The listing builds one solid part. Answer for the finished solid, in the listing's coordinates (mm). A direction names the side the tool comes from. Round coordinates to 2 decimals unless told otherwise and drop trailing zeros. Write each loop counter-clockwise with the first axis right and the second up, starting at its lowest first coordinate (ties: lowest second). Pieces come first, ordered by that corner, then holes. Notation, with made-up numbers: (88, 73.25) - (125, 73.25) arc R21 ccw to (125, 90.25) - close; hole circle Ø1 at (73.25, 44). An arc over 180 degrees is marked (long way). Return JSON: item names as keys, results as strings. Group by question number.
(1) Find the intervals of material crossed by line 1 along Y through (x, z) = (15, 8.25); line 2 along Y through (x, z) = (0, -0.15) (3 decimals); line 3 along Z through (x, y) = (-8.5, 4.25), in increasing order. Write a range as [from, to].
(2) Which of the six approach directions +Z, -Z, +X, -X, +Y, -Y give full straight-line access (tool end or side, diameter ignored) to faces 1 (the cylindrical face through (1.717, -0.541, -0.419)), 2 (the flat face through (9, 7, 0.5)), 3 (the flat face through (-15, 5, -0.001)), 4 (the flat face through (14.5, -5.5, 3.5))?
(3) Each of these flat-tipped pins is pushed along its axis until it touches: pin 1 (6 mm diameter, centred on x = 6, z = 6, fed in from +Y); pin 2 (4 mm diameter, centred on x = 0, y = -0.5, fed in from -Z); pin 3 (6 mm diameter, centred on y = 7.5, z = 0, fed in from +X); pin 4 (1.5 mm diameter, centred on x = -7.5, y = 1, fed in from +Z). Where does it stop, or does it pass through?
(4) Determine the mould class of faces 5 (the flat face through (11, 9, 1)), 6 (the cylindrical face through (1.25, -0.96, 0.59)), 7 (the flat face through (0, 8, 2)) for opening direction X: +X half, -X half, draft (parallel to the pull), parting line (faces both ways), or undercut.
(5) Section A-A, the plane z = 5.25 is taken. Write down the section's boundary in (x, y), then the cut area to 3 significant figures.
(6) Section C-C, the plane x = -13 is taken. Write down the section's boundary in (y, z) (3 decimals), then the cut area to 3 significant figures.
(7) Section B-B, the plane y = 0 is taken. Write down the section's boundary in (x, z) (3 decimals), then the cut area to 3 significant figures.
```python
from build123d import *

# Parameters (mm, degrees)
BOSS_EXTRUDE1_DEPTH     = 2
SKETCH2_R               = 1.575
BOSS_EXTRUDE2_DEPTH     = 4
SKETCH3_R               = 1.8
BOSS_EXTRUDE3_DEPTH     = 0.85
SKETCH4_W               = 2
SKETCH4_H               = 17
BOSS_EXTRUDE4_DEPTH     = 0.001
SKETCH5_W               = 18
SKETCH5_H               = 2
BOSS_EXTRUDE5_DEPTH     = 0.001
SKETCH6_W               = 2.001
SKETCH6_H               = 2
BOSS_EXTRUDE6_DEPTH     = 5
BOSS_EXTRUDE7_DEPTH     = 0.001
CUT_EXTRUDE1_DEPTH      = 20.519323784
SKETCH9_W               = 2.937742252
SKETCH9_H               = 8
CUT_EXTRUDE2_DEPTH      = 0.001
CUT_EXTRUDE11_START     = -0.001
SKETCH21_R              = 9.75
SKETCH21_R_2            = 1.8
CUT_EXTRUDE11_DEPTH     = 0.001
SKETCH10_W              = 32
SKETCH10_H              = 2
BOSS_EXTRUDE8_DEPTH     = 7
FILLET1_R               = 0.5
SKETCH11_R              = 0.625
BOSS_EXTRUDE9_DEPTH     = 2
SKETCH14_W              = 2
SKETCH14_H              = 2
CUT_EXTRUDE5_DEPTH      = 22.401355237
SKETCH12_R              = 0.675
CUT_EXTRUDE3_DEPTH      = 2.5
CUT_EXTRUDE6_DEPTH      = 2
FILLET2_R               = 0.5
FILLET3_R               = 0.5
FILLET4_R               = 2
CUT_EXTRUDE7_DEPTH      = 26.019992106
CUT_EXTRUDE7_DEPTH_BACK = 1
SKETCH19_R              = 0.625
CUT_EXTRUDE9_DEPTH      = 2


with BuildPart() as part:
    # Sketch1 → Boss-Extrude1 (new body)
    with BuildSketch(Plane.XY):
        Polygon((-11, 6), (-11, 11), (11, 11), (11, 6), (11, -6), (-11, -6), align=None)
    extrude(amount=BOSS_EXTRUDE1_DEPTH)

    # Sketch3 → Boss-Extrude3 (add)
    with BuildSketch(Plane(origin=(0, 0, 0), x_dir=(-1, 0, 0), z_dir=(0, 0, -1))):
        with Locations(Location((0, 0, 0), (0, 0, 180))):
            Circle(SKETCH3_R)
    extrude(amount=BOSS_EXTRUDE3_DEPTH)

    # Sketch4 → Boss-Extrude4 (add)
    with BuildSketch(Plane(origin=(0, 0, 0), x_dir=(-1, 0, 0), z_dir=(0, 0, -1))):
        with Locations((10, 2.5)):
            Rectangle(SKETCH4_W, SKETCH4_H)
        with Locations((-10, 2.5)):
            Rectangle(SKETCH4_W, SKETCH4_H)
    extrude(amount=BOSS_EXTRUDE4_DEPTH)

    # Sketch5 → Boss-Extrude5 (add)
    with BuildSketch(Plane(origin=(0, 0, 0), x_dir=(-1, 0, 0), z_dir=(0, 0, -1))):
        with Locations((0, 10)):
            Rectangle(SKETCH5_W, SKETCH5_H)
    extrude(amount=BOSS_EXTRUDE5_DEPTH)

    # Sketch6 → Boss-Extrude6 (add)
    with BuildSketch(Plane(origin=(11, 0, 0), x_dir=(0, 0, -1), z_dir=(1, 0, 0))):
        with Locations((-0.9995, -5)):
            Rectangle(SKETCH6_W, SKETCH6_H)
        with Locations((-0.9995, 5)):
            Rectangle(SKETCH6_W, SKETCH6_H)
    boss_extrude6 = extrude(amount=BOSS_EXTRUDE6_DEPTH)

    # Mirror1: Boss-Extrude6 across plane
    add(boss_extrude6.mirror(Plane(origin=(0, 0, 0), x_dir=(0, 0, 1), z_dir=(1, 0, 0))))

    # Sketch7 → Boss-Extrude7 (add)
    with BuildSketch(Plane(origin=(0, 0, -0.001), x_dir=(-1, 0, 0), z_dir=(0, 0, -1))):
        with BuildLine():
            ThreePointArc((-6.708203932, -6), (-8.407551231, -3.211398808), (-9, 0))
            Line((-9, 0), (-9, -6))
            Line((-9, -6), (-6.708203932, -6))
        make_face()
        with BuildLine():
            Line((-9, 9), (-9, 0))
            ThreePointArc((-9, 0), (-6.363961031, 6.363961031), (0, 9))
            Line((0, 9), (-9, 9))
        make_face()
    boss_extrude7 = extrude(amount=-BOSS_EXTRUDE7_DEPTH)

    # Sketch8 → Cut-Extrude1 (cut, through all)
    with BuildSketch(Plane(origin=(0, 0, -0.001), x_dir=(-1, 0, 0), z_dir=(0, 0, -1))):
        with BuildLine():
            Line((-11, 4), (-9.16515139, 4))
            ThreePointArc((-9.16515139, 4), (-10, 0), (-9.16515139, -4))
            Line((-9.16515139, -4), (-11, -4))
            Line((-11, -4), (-11, 4))
        make_face()
    cut_extrude1 = extrude(amount=-CUT_EXTRUDE1_DEPTH, mode=Mode.SUBTRACT)

    # Sketch9 → Cut-Extrude2 (cut)
    with BuildSketch(Plane(origin=(0, 0, -0.001), x_dir=(-1, 0, 0), z_dir=(0, 0, -1))):
        with Locations((-9.531128874, 0)):
            Rectangle(SKETCH9_W, SKETCH9_H)
    cut_extrude2 = extrude(amount=-CUT_EXTRUDE2_DEPTH, mode=Mode.SUBTRACT)

    # Mirror2: Boss-Extrude7, Cut-Extrude1, Cut-Extrude2 across plane
    add(boss_extrude7.mirror(Plane(origin=(0, 0, 0), x_dir=(0, 0, 1), z_dir=(1, 0, 0))))
    add(cut_extrude1.mirror(Plane(origin=(0, 0, 0), x_dir=(0, 0, 1), z_dir=(1, 0, 0))), mode=Mode.SUBTRACT)
    add(cut_extrude2.mirror(Plane(origin=(0, 0, 0), x_dir=(0, 0, 1), z_dir=(1, 0, 0))), mode=Mode.SUBTRACT)

    # Sketch21 → Cut-Extrude11 (cut)
    with BuildSketch(Plane(origin=(0, 0, -0.001), x_dir=(-1, 0, 0), z_dir=(0, 0, -1)).offset(CUT_EXTRUDE11_START)):
        Circle(SKETCH21_R)
        with Locations(Location((0, 0, 0), (0, 0, 180))):
            Circle(SKETCH21_R_2, mode=Mode.SUBTRACT)
    extrude(amount=CUT_EXTRUDE11_DEPTH, mode=Mode.SUBTRACT)

    # Sketch10 → Boss-Extrude8 (add)
    with BuildSketch(Plane.XY.offset(2)):
        with Locations((0, -5)):
            Rectangle(SKETCH10_W, SKETCH10_H)
        with Locations((0, 5)):
            Rectangle(SKETCH10_W, SKETCH10_H)
    extrude(amount=BOSS_EXTRUDE8_DEPTH)

    # Fillet1
    fillet1_edges = [part.edges().sort_by_distance(p)[0] for p in [
        (10, 0, 2),
        (-10, 0, 2),
    ]]
    fillet(fillet1_edges, radius=FILLET1_R)

    # Sketch11 → Boss-Extrude9 (add)
    with BuildSketch(Plane(origin=(0, 0, -0.001), x_dir=(-1, 0, 0), z_dir=(0, 0, -1))):
        with Locations(Location((-13, -5, 0), (0, 0, 180))):
            Circle(SKETCH11_R)
    boss_extrude9 = extrude(amount=BOSS_EXTRUDE9_DEPTH)

    # Sketch14 → Cut-Extrude5 (cut, through all)
    with BuildSketch(Plane(origin=(0, 0, -0.001), x_dir=(-1, 0, 0), z_dir=(0, 0, -1))):
        with Locations((10, 7)):
            Rectangle(SKETCH14_W, SKETCH14_H)
        with Locations((-10, 7)):
            Rectangle(SKETCH14_W, SKETCH14_H)
    extrude(amount=-CUT_EXTRUDE5_DEPTH, mode=Mode.SUBTRACT)

    # Sketch12 → Cut-Extrude3 (cut)
    with BuildSketch(Plane(origin=(0, 0, -0.001), x_dir=(-1, 0, 0), z_dir=(0, 0, -1))):
        with Locations((13, -5)):
            Circle(SKETCH12_R)
    cut_extrude3 = extrude(amount=-CUT_EXTRUDE3_DEPTH, mode=Mode.SUBTRACT)

    # Sketch16 → Cut-Extrude6 (cut)
    with BuildSketch(Plane(origin=(0, 6, 0), x_dir=(1, 0, 0), z_dir=(0, 1, 0))):
        with BuildLine():
            Line((-9, -1), (-9, -2))
            ThreePointArc((-9, -2), (-8.75, -1.5), (-9, -1))
        make_face()
    cut_extrude6 = extrude(amount=CUT_EXTRUDE6_DEPTH, mode=Mode.SUBTRACT)

    # Mirror3: Boss-Extrude9, Cut-Extrude3 across plane
    add(boss_extrude9.mirror(Plane.ZX))
    add(cut_extrude3.mirror(Plane.ZX), mode=Mode.SUBTRACT)

    # Mirror4: Cut-Extrude6 across plane
    add(cut_extrude6.mirror(Plane(origin=(0, 0, 0), x_dir=(0, 0, 1), z_dir=(1, 0, 0))), mode=Mode.SUBTRACT)

    # Fillet2
    fillet2_edges = [part.edges().sort_by_distance(p)[0] for p in [
        (12.375, -5, -0.001),
        (12.375, 5, -0.001),
    ]]
    fillet(fillet2_edges, radius=FILLET2_R)

    # Fillet3
    # the kernel refuses this fillet: 0.5 mm, written as the material it takes off along each edge
    with BuildSketch(Plane(origin=(-13, -5, -0.001), x_dir=(-1, 0, 0), z_dir=(0, -1, 0))) as fillet3_piece_1:
        with BuildLine():
            CenterArc((0.675 + FILLET3_R, -FILLET3_R), FILLET3_R, 90, 90)
            Line((0.675, -FILLET3_R), (0.675, 0))
            Line((0.675, 0), (0.675 + FILLET3_R, 0))
        make_face()
    revolve(axis=Axis((-13, -5, -0.001), (0, 0, -1)), mode=Mode.SUBTRACT)
    with BuildSketch(Plane(origin=(-13, 5, -0.001), x_dir=(-1, 0, 0), z_dir=(0, 1, 0))) as fillet3_piece_2:
        with BuildLine():
            CenterArc((0.675 + FILLET3_R, FILLET3_R), FILLET3_R, 180, 90)
            Line((0.675, FILLET3_R), (0.675, 0))
            Line((0.675, 0), (0.675 + FILLET3_R, 0))
        make_face()
    revolve(axis=Axis((-13, 5, -0.001), (0, 0, 1)), mode=Mode.SUBTRACT)

    # Fillet4
    fillet4_edges = [part.edges().sort_by_distance(p)[0] for p in [
        (16, -5, 9),
        (-16, -5, 9),
        (-16, 5, 9),
        (16, 5, 9),
    ]]
    fillet(fillet4_edges, radius=FILLET4_R)

    # Sketch17 → Cut-Extrude7 (cut, two sides: drawn at the far end of the back side and taken through both)
    with BuildSketch(Plane.XZ.offset(6).offset(-CUT_EXTRUDE7_DEPTH_BACK)):
        with BuildLine():
            Line((-16, 7), (-16, -0.001))
            Line((-16, -0.001), (-14.5, -0.001))
            Line((-14.5, -0.001), (-14.5, 7))
            ThreePointArc((-14.5, 7), (-14.353553391, 7.353553391), (-14, 7.5))
            Line((-14, 7.5), (14, 7.5))
            ThreePointArc((14, 7.5), (14.353553391, 7.353553391), (14.5, 7))
            Line((14.5, 7), (14.5, -0.001))
            Line((14.5, -0.001), (16, -0.001))
            Line((16, -0.001), (16, 7))
            ThreePointArc((16, 7), (15.414213562, 8.414213562), (14, 9))
            Line((14, 9), (-14, 9))
            ThreePointArc((-14, 9), (-15.414213562, 8.414213562), (-16, 7))
        make_face()
    extrude(amount=CUT_EXTRUDE7_DEPTH + CUT_EXTRUDE7_DEPTH_BACK, mode=Mode.SUBTRACT)

    # Sketch19 → Cut-Extrude9 (cut)
    with BuildSketch(Plane(origin=(0, 6, 0), x_dir=(1, 0, 0), z_dir=(0, 1, 0))):
        with Locations(Location((0, -2.625, 0), (0, 0, 90))):
            Circle(SKETCH19_R)
        with Locations(Location((0, -8.125, 0), (0, 0, 270))):
            Circle(SKETCH19_R)
    extrude(amount=-CUT_EXTRUDE9_DEPTH, mode=Mode.SUBTRACT)


with BuildPart() as body_2:
    # Sketch2 → Boss-Extrude2 (new body)
    with BuildSketch(Plane(origin=(0, 0, 2), x_dir=(-1, 0, 0), z_dir=(0, 0, -1))):
        Circle(SKETCH2_R)
    extrude(amount=BOSS_EXTRUDE2_DEPTH)


with BuildPart() as part_1:
    add(part.part)

    # Combine2: cut body 2
    add(body_2.part, mode=Mode.SUBTRACT)


solid = part_1.part
```
Working result:
{
 "1": {"line 1": "y = [-5, -4], [4, 6]", "line 2": "y = [-1.8, -1.575], [1.575, 1.8]", "line 3": "z = [0, 9]"},
 "2": {"face 1": "-Z", "face 2": "+Z, -Z, +X", "face 3": "-Z, -X, +Y, -Y", "face 4": "+Z, -Z, +X, -Y"},
 "3": {"pin 1": "stops at y = 6", "pin 2": "stops at z = -0.85", "pin 3": "stops at x = 16", "pin 4": "stops at z = 2"},
 "4": {"face 5": "+X half", "face 6": "undercut", "face 7": "draft"},
 "5": {"outline": "(-16, -5) - (-14.5, -5) - (-14.5, -6) - (14.5, -6) - (14.5, -5) - (16, -5) - (16, -4) - (-16, -4) - close; (-16, 4) - (16, 4) - (16, 6) - (-16, 6) - close", "area": "125 mm^2"},
 "6": {"outline": "(-6, 0.031) arc R0.5 ccw to (-5.675, 0.499) - (-5.675, 2.499) - (-4.325, 2.499) - (-4.325, 0.499) arc R0.5 ccw to (-4, 0.031) - (-4, 9) - (-5, 9) - (-5, 7.5) - (-6, 7.5) - close; (4, 0.031) arc R0.5 ccw to (4.325, 0.499) - (4.325, 2.499) - (5.675, 2.499) - (5.675, 0.499) arc R0.5 ccw to (6, 0.031) - (6, 9) - (4, 9) - close", "area": "27.5 mm^2"},
 "7": {"outline": "(-10, 0) - (-1.8, 0) - (-1.8, -0.85) - (-1.575, -0.85) - (-1.575, 2) - (-9.5, 2) arc R0.5 ccw to (-10, 1.5) - close; (1.575, -0.85) - (1.8, -0.85) - (1.8, 0) - (10, 0) - (10, 1.5) arc R0.5 ccw to (9.5, 2) - (1.575, 2) - close", "area": "34.0 mm^2"}
}
